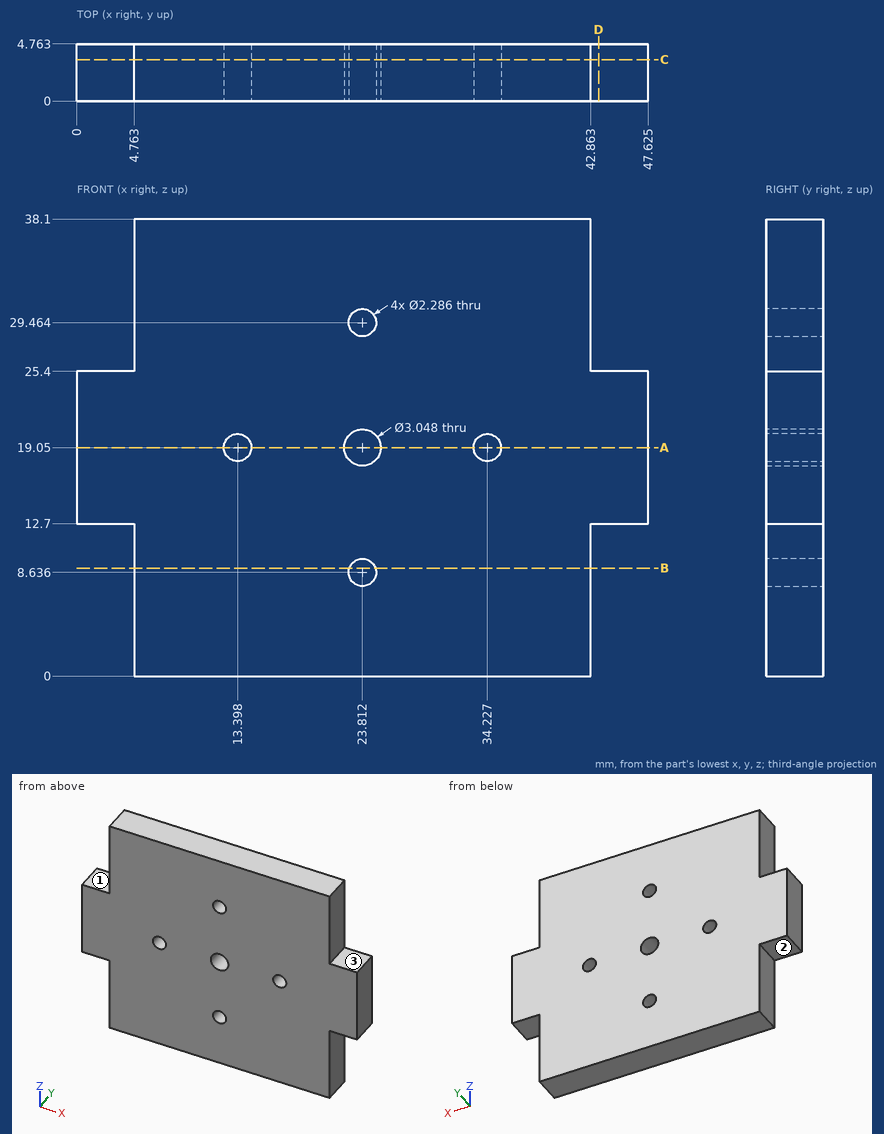
Design review of the part shown in the three views and the two pictorial views. Dimensions are in mm from the part's minimum x, y and z. A direction names the side the tool comes from. Round coordinates to 2 decimals unless told otherwise and drop trailing zeros. Write each loop counter-clockwise with the first axis right and the second up, starting at its lowest first coordinate (ties: lowest second). Pieces come first, ordered by that corner, then holes.
1) Take a section at D-D on x = 43.5. Give the boundary of the cut face in (y, z).
Answer below:
outline: (0, 12.7) - (4.76, 12.7) - (4.76, 25.4) - (0, 25.4) - close
2) Insertion check: pin 1 Ø2.5 at (x, y) = (3, 2.5) entering from -Z; pin 2 Ø2.5 at (x, y) = (46, 2) entering from +Z; pin 3 Ø1.4 at (y, z) = (3.5, 29.5) entering from +X. Each pin has a flat end and moves straight along its axis. Give the tip position at first contact, or say it passes through.
Answer below:
pin 1: stops at z = 12.7
pin 2: stops at z = 25.4
pin 3: stops at x = 42.86
3) Take a section at A-A on z = 19.05. Give the boundary of the cut face in (x, y) (1 decimal).
Answer below:
outline: (0, 0) - (12.3, 0) - (12.3, 4.8) - (0, 4.8) - close; (14.5, 0) - (22.3, 0) - (22.3, 4.8) - (14.5, 4.8) - close; (25.3, 0) - (33.1, 0) - (33.1, 4.8) - (25.3, 4.8) - close; (35.4, 0) - (47.6, 0) - (47.6, 4.8) - (35.4, 4.8) - close
4) Take a section at B-B on z = 9. Give the boundary of the cut face in (x, y) (1 decimal).
Answer below:
outline: (4.8, 0) - (22.7, 0) - (22.7, 4.8) - (4.8, 4.8) - close; (24.9, 0) - (42.9, 0) - (42.9, 4.8) - (24.9, 4.8) - close
5) For line 1 along X through (y, z) = (3.05, 19.05) (1 decimal); line 2 along X through (y, z) = (3.8, 33); line 3 along X through (y, z) = (3.25, 30.5) (1 decimal), list the stretches that pass through material, from the lowest coordinate up.
Answer below:
line 1: x = 0 to 12.3, 14.5 to 22.3, 25.3 to 33.1, 35.4 to 47.6
line 2: x = 4.76 to 42.86
line 3: x = 4.8 to 23.3, 24.3 to 42.9
6) Machinability: for the marked faces 1, 2 and 3, which of the approach directions +Z, -Z, +X, -X, +Y, -Y give a long, thin tool a straight path to every point of the face, cutting with its end or side? Answer none if there is none.
Answer below:
face 1: +Z, -X, +Y, -Y
face 2: -Z, -X, +Y, -Y
face 3: +Z, +X, +Y, -Y
7) Take a section at C-C on y = 3.45. State how many separate pieces and enclosed holes the cut face has, then the cut area to 3 significant figures.
Answer below:
separate pieces: 1
enclosed holes: 5
area: 1,550 mm2
